from build123d import *

# Parameters (mm, degrees)
BOSS_EXTRUDE1_DEPTH = 19
FILLET1_R           = 1.5
FILLET2_R           = 2
FILLET3_R           = 5
CHAMFER1_SIZE       = 0.5


with BuildPart() as part:
    # Sketch1 → Boss-Extrude1 (new body)
    with BuildSketch(Plane(origin=(0, 0, 0), x_dir=(1, 0, 0), z_dir=(0, 1, 0))):
        Polygon((-47.925925926, 24.470420803), (-47.925925926, -7.529579197), (-47.925925926, -22.529579197), (-55.925925926, -22.529579197), (-55.925925926, -25.529579197), (-47.925925926, -25.529579197), (-47.925925926, -28.529579197), (-42.925925926, -28.529579197), (22.074074074, 22.470420803), (22.074074074, 24.470420803), (22.074074074, 27.470420803), (22.074074074, 37.470420803), (17.074074074, 37.470420803), (17.074074074, 27.470420803), (-42.925925926, 27.470420803), (-47.925925926, 27.470420803), (-63.925925926, 27.470420803), (-63.925925926, 24.470420803), (-63.925925926, 19.470420803), (-60.925925926, 19.470420803), (-60.925925926, 24.470420803), align=None)
        Polygon((13.974112284, 22.470420803), (-13.512360238, 0.904111593), (-42.925925926, -22.174224561), (-42.925925926, 22.470420803), align=None, mode=Mode.SUBTRACT)
    extrude(amount=BOSS_EXTRUDE1_DEPTH)

    # Fillet1
    fillet1_edges = [part.edges().sort_by_distance(p)[0] for p in [
        (13.974112284, 9.5, -22.470420803),
        (-42.925925926, 9.5, -22.470420803),
        (-42.925925926, 9.5, 22.174224561),
        (-47.925925926, 9.5, 28.529579197),
        (-55.925925926, 9.5, 25.529579197),
        (-55.925925926, 9.5, 22.529579197),
        (-47.925925926, 9.5, 22.529579197),
        (-63.925925926, 9.5, -27.470420803),
        (-63.925925926, 9.5, -19.470420803),
        (-60.925925926, 9.5, -19.470420803),
        (-42.925925926, 9.5, 28.529579197),
    ]]
    fillet(fillet1_edges, radius=FILLET1_R - 0.0001)  # a hair under: the kernel refuses the full size

    # Fillet2
    fillet2_edges = [part.edges().sort_by_distance(p)[0] for p in [
        (17.074074074, 9.5, -37.470420803),
        (22.074074074, 9.5, -37.470420803),
        (17.074074074, 9.5, -27.470420803),
    ]]
    fillet(fillet2_edges, radius=FILLET2_R)

    # Fillet3
    fillet3_edges = [part.edges().sort_by_distance(p)[0] for p in [
        (22.074074074, 9.5, -22.470420803),
    ]]
    fillet(fillet3_edges, radius=FILLET3_R)

    # Chamfer1
    chamfer1_edges = [part.edges().sort_by_distance(p)[0] for p in [
        (19.574074074, 0, -37.470420803),
        (19.574074074, 19, -37.470420803),
        (17.074074074, 0, -32.470420803),
        (17.659860512, 0, -36.884634365),
        (21.488287636, 0, -36.884634365),
        (17.074074074, 19, -32.470420803),
        (17.659860512, 19, -36.884634365),
        (21.488287636, 19, -36.884634365),
        (16.488287636, 0, -28.056207241),
        (16.488287636, 19, -28.056207241),
        (22.074074074, 0, -30.186559659),
        (22.074074074, 19, -30.186559659),
        (-11.178869129, 0, 3.620350018),
        (21.570304248, 0, -22.715482427),
        (-11.178869129, 19, 3.620350018),
        (21.570304248, 19, -22.715482427),
        (-47.925925926, 0, 26.279629197),
        (-54.425925926, 0, -24.470420803),
        (-60.925925926, 0, -22.720370803),
        (-60.925925926, 19, -22.720370803),
        (-54.425925926, 19, -24.470420803),
        (-44.935070567, 0, 28.529579197),
        (-47.925925926, 19, 26.279629197),
        (-51.175975926, 0, 25.529579197),
        (-51.925925926, 0, 22.529579197),
        (-47.925925926, 0, -1.720370803),
        (-63.925925926, 0, -23.470420803),
        (-23.675975926, 0, -27.470420803),
        (-42.925925926, 0, -0.93981007),
        (-14.970820153, 0, 0.240218493),
        (-15.896688718, 0, -22.470420803),
        (-61.365236465, 0, -19.909731342),
        (-63.486615387, 0, -19.909731342),
        (-63.486615387, 0, -27.031110264),
        (-55.486615387, 0, 22.968889736),
        (-55.486615387, 0, 25.090268658),
        (-47.486615387, 0, 28.090268658),
        (-42.954332008, 0, 28.447357731),
        (-44.935070567, 19, 28.529579197),
        (-23.675975926, 19, -27.470420803),
        (-63.925925926, 19, -23.470420803),
        (-47.925925926, 19, -1.720370803),
        (-51.925925926, 19, 22.529579197),
        (-51.175975926, 19, 25.529579197),
        (-42.925925926, 19, -0.93981007),
        (-15.896688718, 19, -22.470420803),
        (-14.970820153, 19, 0.240218493),
        (-61.365236465, 19, -19.909731342),
        (-63.486615387, 19, -19.909731342),
        (-63.486615387, 19, -27.031110264),
        (-55.486615387, 19, 22.968889736),
        (-55.486615387, 19, 25.090268658),
        (-47.486615387, 19, 28.090268658),
        (-42.954332008, 19, 28.447357731),
        (11.050327025, 0, -21.460304004),
        (11.050327025, 19, -21.460304004),
        (-42.486615387, 0, -22.031110264),
        (-42.486615387, 19, -22.031110264),
        (-42.082147008, 0, 20.43967979),
        (-42.082147008, 19, 20.43967979),
        (-48.365236465, 0, 22.090268658),
        (-48.365236465, 19, 22.090268658),
    ]]
    chamfer(chamfer1_edges, length=CHAMFER1_SIZE)


solid = part.part
The listing builds one solid part. Answer for the finished solid, in the listing's coordinates (mm). A direction names the side the tool comes from. Round coordinates to 2 decimals unless told otherwise and drop trailing zeros. Write each loop counter-clockwise with the first axis right and the second up, starting at its lowest first coordinate (ties: lowest second). Pieces come first, ordered by that corner, then holes. Notation, with made-up numbers: (76, 3) - (129, 3) arc R24 cw to (129, 20) - close; hole circle Ø7 at (46, -17.75). An arc over 180 degrees is marked (long way). Use a Markdown table: item, result. Add a question column.
1. The part is cut by section C-C (z = 5). Write down the section's boundary in (x, y).
2. For a pull along X with two mould halves and no side action, classify faces 5 (the face through (11.169, 0.365, -21.531)), 6 (the face through (21.58, 9.63, -22.74)), 7 (the face through (17.644, 9.626, -36.869)), 8 (the face through (-52, 9, 22.53)) as +X half, -X half, draft (parallel to the pull), parting line (faces both ways), or undercut.
3. Consider line 1 (X direction, y = 9.75, z = -20); line 2 (Z direction, x = -51, y = 16); line 3 (Z direction, x = -19.5, y = 10.25). Determine where each line is inside the solid, lowest interval first.
4. A tool of negligible diameter and unlimited length cuts with its end or side. For faces 1 (the face through (-42.595, 0.365, -22.114)), 2 (the face through (-23, 9, -27.47)), 3 (the face through (-16, 9, -22.47)), 4 (the face through (-42.121, 18.642, 20.579)), from which of +Z, -Z, +X, -X, +Y, -Y can it reach the whole face along a straight path? Write none if from no direction.
5. Flat-ended cylindrical pins translate along their axes: P1, Ø9, axis at y = 11.5, z = 7, coming from the +X side; P2, Ø5.5, axis at x = -30.5, y = 5.5, coming from the -Z side; P3, Ø5.5, axis at x = -5, y = 5, coming from the +Z side; P4, Ø12, axis at x = -2, z = -13, coming from the -Y side. Find the tip coordinate at first contact, or state that the pin passes through.
6. The part is cut by section A-A (x = -53.5). Write down the section's boundary in (y, z).
Reported:
| question | item | result |
|---|---|---|
| 1 | outline | (-47.93, 0.5) - (-47.43, 0) - (-43.43, 0) - (-42.93, 0.5) - (-42.93, 18.5) - (-43.43, 19) - (-47.43, 19) - (-47.93, 18.5) - close; (-21.04, 0.5) - (-20.23, 0) - (-13.75, 0) - (-12.94, 0.5) - (-12.94, 18.5) - (-13.75, 19) - (-20.23, 19) - (-21.04, 18.5) - close |
| 2 | face 5 | undercut |
| 2 | face 6 | +X half |
| 2 | face 7 | -X half |
| 2 | face 8 | draft |
| 3 | line 1 | -63.57 to -61.28, -47.93 to -42.93, 10.78 to 18.93 |
| 3 | line 2 | -27.47 to -24.47, 22.53 to 25.53 |
| 3 | line 3 | -27.47 to -22.47, 3.79 to 10.15 |
| 4 | face 1 | -Y |
| 4 | face 2 | -Z, -X, +Y, -Y |
| 4 | face 3 | +Y, -Y |
| 4 | face 4 | +Y |
| 5 | P1 | x = -9.75 |
| 5 | P2 | z = -27.47 |
| 5 | P3 | z = 0.93 |
| 5 | P4 | y = 0 |
| 6 | outline | (0, -26.97) - (0.5, -27.47) - (18.5, -27.47) - (19, -26.97) - (19, -24.97) - (18.5, -24.47) - (0.5, -24.47) - (0, -24.97) - close; (0, 23.03) - (0.5, 22.53) - (18.5, 22.53) - (19, 23.03) - (19, 25.03) - (18.5, 25.53) - (0.5, 25.53) - (0, 25.03) - close |
